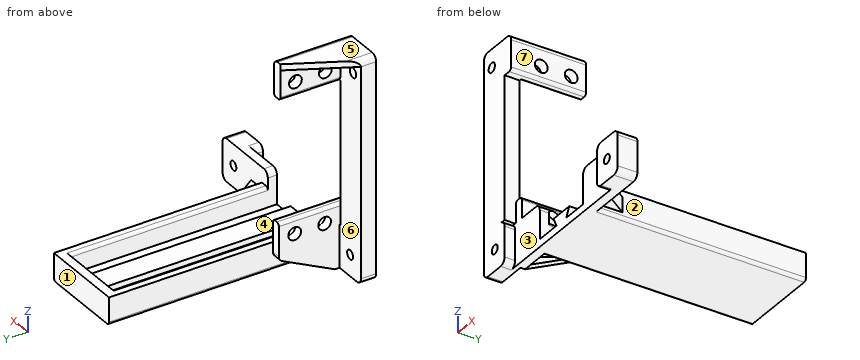
from build123d import *

# Parameters (mm, degrees)
SKETCH_1_W          = 28
SKETCH_1_H          = 14
SKETCH_1_W_2        = 22
SKETCH_1_H_2        = 8
EXTRUDE_1_DEPTH     = 75
SKETCH_2_W          = 22
SKETCH_2_H          = 8
EXTRUDE_2_DEPTH     = 3
SKETCH_3_W          = 22
SKETCH_3_H          = 11
CUT_EXTRUDE_1_DEPTH = 72
SKETCH_4_W          = 20
SKETCH_4_H          = 14
EXTRUDE_3_DEPTH     = 6.5
SKETCH_5_R          = 1.5
CUT_EXTRUDE_2_DEPTH = 83.643814046
FILLET_1_R          = 2
EXTRUDE_5_REACH     = 84.644
SKETCH_9_W          = 28
SKETCH_9_H          = 5
CUT_EXTRUDE_3_DEPTH = 68.5
FILLET_3_R          = 1
EXTRUDE_6_DEPTH     = 2.5
SKETCH_11_W         = 12
SKETCH_11_H         = 25
SKETCH_11_R         = 2.1
EXTRUDE_7_DEPTH     = 3
EXTRUDE_9_DEPTH     = 3
EXTRUDE_8_DEPTH     = 3
SKETCH_16_W         = 47
SKETCH_16_H         = 24
CUT_EXTRUDE_4_DEPTH = 3.5
FILLET_12_R         = 2
FILLET_14_R         = 2
SKETCH_17_W         = 10.5
SKETCH_17_H         = 5
EXTRUDE_10_DEPTH    = 58.7
SKETCH_18_W         = 11.8
SKETCH_18_H         = 24.7
EXTRUDE_11_DEPTH    = 3.35
CUT_EXTRUDE_5_REACH = 115.462
SKETCH_19_R         = 2.1
CUT_EXTRUDE_6_REACH = 103.845
SKETCH_20_R         = 1.6
CUT_EXTRUDE_7_REACH = 103.127
SKETCH_21_W         = 10.85
SKETCH_21_H         = 1.5
EXTRUDE_12_DEPTH    = 2
FILLET_15_R         = 2
FILLET_16_R         = 1
CUT_EXTRUDE_8_DEPTH = 68.5


with BuildPart() as part:
    # 草图1 → 凸台-拉伸1 (new body)
    with BuildSketch(Plane(origin=(0, 0, 0), x_dir=(1, 0, 0), z_dir=(0, 1, 0))):
        Rectangle(SKETCH_1_W, SKETCH_1_H)
        Rectangle(SKETCH_1_W_2, SKETCH_1_H_2, mode=Mode.SUBTRACT)
    extrude(amount=EXTRUDE_1_DEPTH)

    # 草图2 → 凸台-拉伸2 (add)
    with BuildSketch(Plane(origin=(0, 75, 0), x_dir=(1, 0, 0), z_dir=(0, 1, 0))):
        Rectangle(SKETCH_2_W, SKETCH_2_H)
    extrude(amount=-EXTRUDE_2_DEPTH)

    # 草图3 → 切除-拉伸1 (cut)
    with BuildSketch(Plane.XZ):
        with Locations((0, 1.5)):
            Rectangle(SKETCH_3_W, SKETCH_3_H)
    extrude(amount=-CUT_EXTRUDE_1_DEPTH, mode=Mode.SUBTRACT)

    # 草图4 → 凸台-拉伸3 (add)
    with BuildSketch(Plane.XZ):
        with Locations((-24, 0)):
            Rectangle(SKETCH_4_W, SKETCH_4_H)
        with Locations((24, 0)):
            Rectangle(SKETCH_4_W, SKETCH_4_H)
    extrude(amount=-EXTRUDE_3_DEPTH)

    # 草图5 → 切除-拉伸2 (cut, through all)
    with BuildSketch(Plane.XZ):
        with Locations(Location((-28.5, 0, 0), (0, 0, 270))):
            Circle(SKETCH_5_R)
        with Locations(Location((28.5, 0, 0), (0, 0, 270))):
            Circle(SKETCH_5_R)
    extrude(amount=-CUT_EXTRUDE_2_DEPTH, mode=Mode.SUBTRACT)

    # 圆角1
    fillet_1_edges = [part.edges().sort_by_distance(p)[0] for p in [
        (-34, 3.25, -7),
        (34, 3.25, 7),
        (34, 3.25, -7),
    ]]
    fillet(fillet_1_edges, radius=FILLET_1_R)

    # 草图7 → 凸台-拉伸5 (add, up to next)
    with BuildSketch(Plane.XZ, mode=Mode.PRIVATE) as extrude_5_sk1:
        Polygon((-2.5, -4.5), (2.5, -4.5), (4, -1.5), (-4, -1.5), align=None)
    extrude_5_tool1 = extrude(extrude_5_sk1.sketch, amount=-EXTRUDE_5_REACH, mode=Mode.PRIVATE) - part.part
    add(extrude_5_tool1.solids().sort_by_distance((0, 0, -2.884615))[0])

    # 草图9 → 切除-拉伸3 (cut)
    with BuildSketch(Plane(origin=(0, 75, 0), x_dir=(1, 0, 0), z_dir=(0, 1, 0))):
        with Locations((0, -4.5)):
            Rectangle(SKETCH_9_W, SKETCH_9_H)
    extrude(amount=-CUT_EXTRUDE_3_DEPTH, mode=Mode.SUBTRACT)

    # 圆角3
    fillet_3_edges = [part.edges().sort_by_distance(p)[0] for p in [
        (11, 39.25, 2),
        (-11, 39.25, 2),
        (-14, 40.75, -7),
        (14, 40.75, -7),
    ]]
    fillet(fillet_3_edges, radius=FILLET_3_R)

    # 草图10 → 凸台-拉伸6 (add, symmetric)
    with BuildSketch(Plane(origin=(0, 0, -2.5), x_dir=(-1, 0, 0), z_dir=(0, 0, -1))):
        Polygon((-14, 6.5), (-19.5, 6.5), (-14, 14.5), align=None)
    extrude_6 = extrude(amount=EXTRUDE_6_DEPTH, both=True)

    # 镜向2: 凸台-拉伸6 across plane
    add(extrude_6.mirror(Plane(origin=(0, 0, 0), x_dir=(0, 0, 1), z_dir=(1, 0, 0))))

    # 草图11 → 凸台-拉伸7 (add)
    with BuildSketch(Plane.ZY.offset(20.15)):
        with Locations((8, 12.5)):
            Rectangle(SKETCH_11_W, SKETCH_11_H)
        with Locations((8.988854382, 19.775)):
            Circle(SKETCH_11_R, mode=Mode.SUBTRACT)
        with Locations((8.988854382, 9.925)):
            Circle(SKETCH_11_R, mode=Mode.SUBTRACT)
    extrude(amount=EXTRUDE_7_DEPTH)

    # 草图14 → 凸台-拉伸9 (add)
    with BuildSketch(Plane.ZY.offset(23.15)):
        Polygon((2, 25), (-7, 6.5), (2, 6.5), align=None)
    extrude(amount=-EXTRUDE_9_DEPTH)

    # 草图12 → 凸台-拉伸8 (add)
    with BuildSketch(Plane.XY.offset(7)):
        Polygon((-20.15, 6.5), (-20.15, 25), (-11, 6.5), align=None)
    extrude(amount=-EXTRUDE_8_DEPTH)

    # 草图16 → 切除-拉伸4 (cut)
    with BuildSketch(Plane.XZ):
        with Locations((0, 5)):
            Rectangle(SKETCH_16_W, SKETCH_16_H)
    extrude(amount=-CUT_EXTRUDE_4_DEPTH, mode=Mode.SUBTRACT)

    # 圆角12
    fillet_12_edges = [part.edges().sort_by_distance(p)[0] for p in [
        (-11, 5, 7),
        (11, 5, 7),
        (-23.5, 1.75, 7),
        (-23.5, 1.75, -7),
        (23.5, 1.75, 7),
        (23.5, 1.75, -7),
    ]]
    fillet(fillet_12_edges, radius=FILLET_12_R)

    # 圆角14
    fillet_14_edges = [part.edges().sort_by_distance(p)[0] for p in [
        (-21.65, 25, 2),
    ]]
    fillet(fillet_14_edges, radius=FILLET_14_R)

    # 草图17 → 凸台-拉伸10 (add)
    with BuildSketch(Plane.XY.offset(7)):
        with Locations((-28.75, 2.5)):
            Rectangle(SKETCH_17_W, SKETCH_17_H)
    extrude(amount=EXTRUDE_10_DEPTH)

    # 草图18 → 凸台-拉伸11 (add)
    with BuildSketch(Plane(origin=(-23.5, 0, 0), x_dir=(0, 0, -1), z_dir=(1, 0, 0))):
        with Locations((-59.8, 12.35)):
            Rectangle(SKETCH_18_W, SKETCH_18_H)
    extrude(amount=EXTRUDE_11_DEPTH)

    # 草图19 → 切除-拉伸5 (cut, up to next)
    with BuildSketch(Plane(origin=(-20.15, 0, 0), x_dir=(0, 0, -1), z_dir=(1, 0, 0)), mode=Mode.PRIVATE) as cut_extrude_5_sk1:
        with Locations(Location((-58.411145618, 9.925, 0), (0, 0, 90))):
            Circle(SKETCH_19_R)
    cut_extrude_5_tool1 = extrude(cut_extrude_5_sk1.sketch, amount=-CUT_EXTRUDE_5_REACH, mode=Mode.PRIVATE) & part.part
    # 草图19 → 切除-拉伸5 (cut, up to next)
    with BuildSketch(Plane(origin=(-20.15, 0, 0), x_dir=(0, 0, -1), z_dir=(1, 0, 0)), mode=Mode.PRIVATE) as cut_extrude_5_sk2:
        with Locations(Location((-58.411145618, 19.775, 0), (0, 0, 90))):
            Circle(SKETCH_19_R)
    cut_extrude_5_tool2 = extrude(cut_extrude_5_sk2.sketch, amount=-CUT_EXTRUDE_5_REACH, mode=Mode.PRIVATE) & part.part
    add(cut_extrude_5_tool1.solids().sort_by_distance((-20.15, 9.925, 58.411146))[0], mode=Mode.SUBTRACT)
    add(cut_extrude_5_tool2.solids().sort_by_distance((-20.15, 19.775, 58.411146))[0], mode=Mode.SUBTRACT)

    # 草图20 → 切除-拉伸6 (cut, up to next)
    with BuildSketch(Plane(origin=(0, 5, 0), x_dir=(1, 0, 0), z_dir=(0, 1, 0)), mode=Mode.PRIVATE) as cut_extrude_6_sk1:
        with Locations(Location((-30, -59.7, 0), (0, 0, 270))):
            Circle(SKETCH_20_R)
    cut_extrude_6_tool1 = extrude(cut_extrude_6_sk1.sketch, amount=-CUT_EXTRUDE_6_REACH, mode=Mode.PRIVATE) & part.part
    add(cut_extrude_6_tool1.solids().sort_by_distance((-30, 5, 59.7))[0], mode=Mode.SUBTRACT)

    # 草图21 → 切除-拉伸7 (cut, up to next)
    with BuildSketch(Plane.XY.offset(7), mode=Mode.PRIVATE) as cut_extrude_7_sk1:
        with Locations((-28.575, 5.75)):
            Rectangle(SKETCH_21_W, SKETCH_21_H)
    cut_extrude_7_tool1 = extrude(cut_extrude_7_sk1.sketch, amount=-CUT_EXTRUDE_7_REACH, mode=Mode.PRIVATE) & part.part
    add(cut_extrude_7_tool1.solids().sort_by_distance((-28.575, 5.75, 7))[0], mode=Mode.SUBTRACT)

    # 草图22 → 凸台-拉伸12 (add)
    with BuildSketch(Plane.XY.offset(65.7)):
        Polygon((-23.5, 5), (-34, 5), (-23.5, 24.7), align=None)
    extrude(amount=-EXTRUDE_12_DEPTH)

    # 圆角15
    fillet_15_edges = [part.edges().sort_by_distance(p)[0] for p in [
        (-34, 2.5, 65.7),
        (-20.15, 12.35, 65.7),
    ]]
    fillet(fillet_15_edges, radius=FILLET_15_R)

    # 圆角16
    fillet_16_edges = [part.edges().sort_by_distance(p)[0] for p in [
        (-20.15, 14.25, 14),
        (-23.15, 14.25, 14),
        (-23.5, 14.85, 53.9),
        (-20.15, 12.35, 53.9),
    ]]
    fillet(fillet_16_edges, radius=FILLET_16_R)

    # 草图23 → 切除-拉伸8 (cut)
    with BuildSketch(Plane.XZ.offset(-3.5)):
        Polygon((-11, -4), (-11, -4.5), (-2.5, -4.5), (-2.75, -4), align=None)
        Polygon((11, -4), (11, -4.5), (2.5, -4.5), (2.75, -4), align=None)
    extrude(amount=-CUT_EXTRUDE_8_DEPTH, mode=Mode.SUBTRACT)


solid = part.part
Input: part model. Units: mm. Frame: model coordinates. Face numbers are marked on the shaded views. A direction names the side the tool comes from. Coordinates: 2 decimals unless noted, no trailing zeros. Loops run counter-clockwise (first coordinate to the right, second up) from the corner with the lowest first, then second, coordinate; pieces in that order, holes last. Notation, with made-up numbers: (78.5, 36.5) -> (97.5, 36.5) arc R14 cw to (97.5, 40.5) -> close; hole circle Ø10 at (-14, 46). An arc over 180 degrees is marked (long way). Write item = value, one per line. Start each with the question number.
Item 1: Mould query, pull axis X, two halves, no side actions, for the marked faces 1, 2, 3 and 4. Classes: pulls with the +X half, pulls with the -X half, needs draft (parallel to the pull), parting line crosses it, or undercut.
Item 2: First-contact query: P1, Ø6, axis at x = 4, y = 25.5, coming from the +Z side; P2, Ø22.5, axis at x = -5, y = 52.5, coming from the +Z side; P3, Ø6, axis at x = -22, y = 13.5, coming from the +Z side; P4, Ø1.7, axis at x = -22.5, z = 57.5, coming from the +Y side. Flat tips, straight axial feed; report the tip coordinate or a pass-through.
Item 3: Material intervals for line 1 (X direction, y = 3, z = 59.7); line 2 (X direction, y = 2, z = 0); line 3 (Z direction, x = -20, y = 5), sorted ascending.
Item 4: Reachability of the marked faces 5, 6 and 7 from +Z, -Z, +X, -X, +Y, -Y: full face, straight path, thin tool, end or side. Return the list, or none.
Item 5: Cut plane B-B, the plane y = 65. Return loops of the section in (x, z).
Item 6: Cut plane C-C, the plane x = -6.5. Return loops of the section in (y, z), plus the area to 3 significant figures.
Item 7: Cut plane A-A, the plane x = 28.5. Return loops of the section in (y, z).
Item 8: Cut plane D-D, the plane z = 38.5. Return loops of the section in (x, y).
Ans:
q1.face_1 = needs draft
q1.face_2 = pulls with the +X half
q1.face_3 = undercut
q1.face_4 = undercut
q2.P1 = -1.5
q2.P2 = 2
q2.P3 = 65.7
q2.P4 = 24.7
q3.line_1 = -34 to -31.6, -28.4 to -20.15
q3.line_2 = -34 to -30, -27 to -23.5, 23.5 to 27, 30 to 34
q3.line_3 = -7 to 7
q4.face_5 = +Z, +X, -X, +Y, -Y
q4.face_6 = -Z, -X, +Y
q4.face_7 = +Z, +X, +Y, -Y
q5.outline = (-14, -6) arc R1 ccw to (-13, -7) -> (13, -7) arc R1 ccw to (14, -6) -> (14, 2) -> (12, 2) arc R1 ccw to (11, 1) -> (11, -4.5) -> (2.5, -4.5) -> (4, -1.5) -> (-4, -1.5) -> (-2.5, -4.5) -> (-11, -4.5) -> (-11, 1) arc R1 ccw to (-12, 2) -> (-14, 2) -> close
q6.outline = (3.5, -7) -> (75, -7) -> (75, 2) -> (72, 2) -> (72, -4.5) -> (3.5, -4.5) -> close
q6.area = 198 mm²
q7.outline = (0, -7) -> (6.5, -7) -> (6.5, -1.5) -> (0, -1.5) -> close; (0, 1.5) -> (6.5, 1.5) -> (6.5, 7) -> (0, 7) -> close
q8.outline = (-34, 0) -> (-23.5, 0) -> (-23.5, 5) -> (-34, 5) -> close
